Can you work these out from the model? Positions are in its coordinate system, mm. Face numbers are marked on the shaded views. A direction names the side the tool comes from. Coordinates: 2 decimals unless noted, no trailing zeros. Loops run counter-clockwise (first coordinate to the right, second up) from the corner with the lowest first, then second, coordinate; pieces in that order, holes last.
```python
from build123d import *

# Parameters (mm, degrees)
SKETCH1_W                    = 140
SKETCH1_H                    = 140
BASE_FLANGE1_DEPTH           = 2
EDGE_FLANGE2_STRIP_W         = 9.4732
EDGE_FLANGE2_STRIP_H         = 2
EDGE_FLANGE2_STRIP_CUT_DEPTH = 140
EDGE_FLANGE2_DEPTH           = 140
EDGE_FLANGE3_STRIP_W         = 9.4732
EDGE_FLANGE3_STRIP_H         = 2
EDGE_FLANGE3_STRIP_CUT_DEPTH = 140
EDGE_FLANGE3_DEPTH           = 140


# Sheet-metal steps are written as plain solids
with BuildPart() as part:
    # Sketch1 → Base-Flange1 (new body)
    with BuildSketch(Plane(origin=(0, 0, 0), x_dir=(1, 0, 0), z_dir=(0, 1, 0))):
        with Locations((-8.720538721, -25.533108866)):
            Rectangle(SKETCH1_W, SKETCH1_H)
    extrude(amount=-BASE_FLANGE1_DEPTH)

    # Edge-Flange2 strip (across the edge) → Edge-Flange2 strip cut (cut)
    with BuildSketch(Plane(origin=(-78.720538721, 0, 95.533108866), x_dir=(0, 0, -1), z_dir=(1, 0, 0))):
        with Locations((-2, -1)):
            Rectangle(EDGE_FLANGE2_STRIP_W, EDGE_FLANGE2_STRIP_H)
    extrude(amount=EDGE_FLANGE2_STRIP_CUT_DEPTH, mode=Mode.SUBTRACT)

    # Edge-Flange2 section (across the edge) → Edge-Flange2 (add)
    with BuildSketch(Plane(origin=(-78.720538721, 0, 95.533108866), x_dir=(0, 0, -1), z_dir=(1, 0, 0))):
        with BuildLine():
            Line((0, 0.7366), (0, 278))
            Line((0, 278), (2, 278))
            Line((2, 278), (2, 0.7366))
            ThreePointArc((2, 0.7366), (2.215745145, 0.215745145), (2.7366, 0))
            Line((2.7366, 0), (2.7366, -2))
            ThreePointArc((2.7366, -2), (0.801531583, -1.198468417), (0, 0.7366))
        make_face()
    extrude(amount=EDGE_FLANGE2_DEPTH)

    # Edge-Flange3 strip (across the edge) → Edge-Flange3 strip cut (cut)
    with BuildSketch(Plane(origin=(-78.720538721, 278, 93.533108866), x_dir=(0, -1, 0), z_dir=(1, 0, 0))):
        with Locations((-2, -1)):
            Rectangle(EDGE_FLANGE3_STRIP_W, EDGE_FLANGE3_STRIP_H)
    extrude(amount=EDGE_FLANGE3_STRIP_CUT_DEPTH, mode=Mode.SUBTRACT)

    # Edge-Flange3 section (across the edge) → Edge-Flange3 (add)
    with BuildSketch(Plane(origin=(-78.720538721, 278, 93.533108866), x_dir=(0, -1, 0), z_dir=(1, 0, 0))):
        with BuildLine():
            Line((0, 0.7366), (0, 48))
            Line((0, 48), (2, 48))
            Line((2, 48), (2, 0.7366))
            ThreePointArc((2, 0.7366), (2.215745145, 0.215745145), (2.7366, 0))
            Line((2.7366, 0), (2.7366, -2))
            ThreePointArc((2.7366, -2), (0.801531583, -1.198468417), (0, 0.7366))
        make_face()
    extrude(amount=EDGE_FLANGE3_DEPTH)


solid = part.part
```
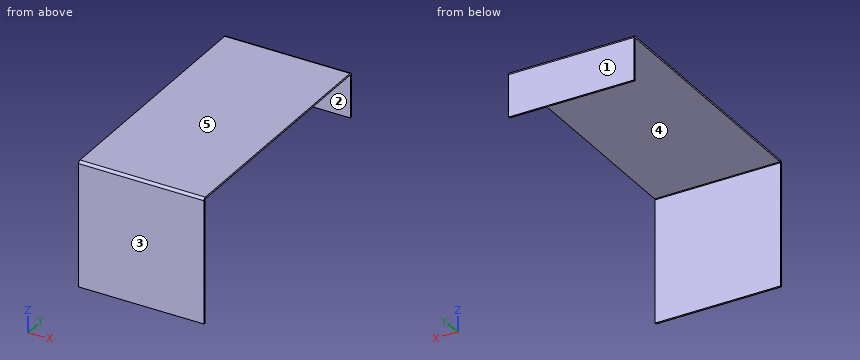
(1) I'm going to push flat-ended pins straight in: pin 1 (2 mm diameter, centred on x = -7.5, y = 164, fed in from -Z); pin 2 (0.6 mm diameter, centred on x = -9, y = 276.5, fed in from -Z). Where does each tip first touch, or does it pass through?
Check values:
pin 1: stops at z = 93.53
pin 2: stops at z = 45.53
(2) I want a section at B-B on x = -35.5. Write out the boundary of the cut face in (y, z).
Check values:
outline: (-2, -44.47) - (0, -44.47) - (0, 92.8) arc R0.74 cw to (0.74, 93.53) - (275.26, 93.53) arc R0.74 cw to (276, 92.8) - (276, 45.53) - (278, 45.53) - (278, 92.8) arc R2.74 ccw to (275.26, 95.53) - (0.74, 95.53) arc R2.74 ccw to (-2, 92.8) - close
(3) I want a section at A-A on z = 79. Write out the boundary of the cut face in (x, y).
Check values:
outline: (-78.72, -2) - (61.28, -2) - (61.28, 0) - (-78.72, 0) - close; (-78.72, 276) - (61.28, 276) - (61.28, 278) - (-78.72, 278) - close
(4) Which directions (+Z, -Z, +X, -X, +Y, -Y) give clear straight access to the entire face, cutting with the end or side of a thin tool? Please do the marked faces 4 and 5.
Check values:
face 4: -Z, +X, -X
face 5: +Z, +X, -X, +Y, -Y
(5) If we mould it in two halves opening along Y, with no side actions, what happens to the marked faces 1, 2 and 3? For each: released by +Y, released by -Y, zero draft, split by the parting line, or undercut.
Check values:
face 1: released by +Y
face 2: undercut
face 3: released by -Y
(6) If I drill on probe 1 along Y at (x, z) = (55.5, 66); probe 2 along Z at (x, y) = (38, 101.5); probe 3 along Y at (x, z) = (2.5, -9), over which ranges is the centre line in solid material (lowest first)?
Check values:
probe 1: y = -2 to 0, 276 to 278
probe 2: z = 93.53 to 95.53
probe 3: y = -2 to 0
(7) I want a section at D-D on z = -16. Write out the boundary of the cut face in (x, y), then the cut area to 3 significant figures.
Check values:
outline: (-78.72, -2) - (61.28, -2) - (61.28, 0) - (-78.72, 0) - close
area: 280 mm2
(8) I want a section at C-C on y = 145. Write out the boundary of the cut face in (x, z), then the cut area to 3 significant figures.
Check values:
outline: (-78.72, 93.53) - (61.28, 93.53) - (61.28, 95.53) - (-78.72, 95.53) - close
area: 280 mm2
